Check sheet for the modelled part. Datum: model origin and axes. Units: mm. A direction names the side the tool comes from. Round coordinates to 2 decimals unless told otherwise and drop trailing zeros. Write each loop counter-clockwise with the first axis right and the second up, starting at its lowest first coordinate (ties: lowest second). Pieces come first, ordered by that corner, then holes.
Item 1: Section check A-A, the plane x = -7.75. Record the cut outline in (y, z).
Item 2: Release check for a two-part mould opening along X. For faces 1 (the cylindrical face through (-14.1, 49.3, 14.14)), 2 (the flat face through (0, 49, 13)), 3 (the flat face through (14, 0, 0)), 4 (the cylindrical face through (14.1, 49.3, -14.14)) record: pulls with the +X half, pulls with the -X half, needs draft (parallel to the pull), parting line crosses it, or undercut.
Item 3: Section check B-B, the plane z = 4.5. Record the cut outline in (x, y).
Item 4: Material ranges on line 1 along X through (y, z) = (61.5, 7.5); line 2 along Z through (x, y) = (12.5, 78), recorded low to high.
Item 5: Set-up check for faces 5 (the flat face through (0, 49, 15)), 6 (the flat face through (-13, 49, 0)): record each of +Z, -Z, +X, -X, +Y, -Y from which the full face is reachable in a straight line by a thin tool's end or side.
Item 6: Section check C-C, the plane y = 87. Record the cut outline in (x, z), plus the area to 3 significant figures.
Autodesk Inventor part; units mm, degrees
ref_plane "YZ Plane" through (0, 0, 0) normal (1, 0, 0) x (0, 1, 0)
ref_plane "XZ Plane" through (0, 0, 0) normal (0, 1, 0) x (-1, 0, 0)
ref_plane "XY Plane" through (0, 0, 0) normal (0, 0, 1) x (1, 0, 0)
sketch "Sketch1" plane through (0, 0, 0) normal (0, 1, 0) x (-1, 0, 0)
  line L0 (-12, 14) -> (12, 14) construction
  line L1 (14, 12) -> (14, -12) construction
  line L2 (12, -14) -> (-12, -14) construction
  line L3 (-14, -12) -> (-14, 12) construction
  line L4 (-14, 14) -> (14, -14) construction
  line L5 (14, 14) -> (-14, -14) construction
  arc A0 (14, 12) -> (12, 14) centre (12, 12) ccw construction
  arc A1 (12, -14) -> (14, -12) centre (12, -12) ccw construction
  arc A2 (-14, -12) -> (-12, -14) centre (-12, -12) ccw construction
  arc A3 (-12, 14) -> (-14, 12) centre (-12, 12) ccw construction
  line L6 (-12, -15) -> (12, -15)
  arc A4 (12, -15) -> (15, -12) centre (12, -12) ccw
  line L7 (15, -12) -> (15, 12)
  arc A5 (15, 12) -> (12, 15) centre (12, 12) ccw
  line L8 (12, 15) -> (-12, 15)
  arc A6 (-12, 15) -> (-15, 12) centre (-12, 12) ccw
  line L9 (-15, 12) -> (-15, -12)
  arc A7 (-15, -12) -> (-12, -15) centre (-12, -12) ccw
  line L10 (13, -12) -> (13, 12)
  arc A8 (13, 12) -> (12, 13) centre (12, 12) ccw
  line L11 (12, 13) -> (-12, 13)
  arc A9 (-12, 13) -> (-13, 12) centre (-12, 12) ccw
  line L12 (-13, 12) -> (-13, -12)
  arc A10 (-13, -12) -> (-12, -13) centre (-12, -12) ccw
  line L13 (-12, -13) -> (12, -13)
  arc A11 (12, -13) -> (13, -12) centre (12, -12) ccw
  point P0 (0, 0)
  point P1 (0, 0)
  point P2 (0, 0)
  dimension "d10" = 2
  dimension "depth" = 30
  dimension "width" = 30
  dimension "thickness" = 2
extrude "Extrusion1" add sketch "Sketch1" along normal blind 100
equation "\"d10\" = thickness"
properties part number "beam 30x30x2" material "Steel"
Values found:
1. outline: (0, -15) - (100, -15) - (100, -13) - (0, -13) - close; (0, 13) - (100, 13) - (100, 15) - (0, 15) - close
2. face 1: pulls with the -X half
2. face 2: undercut
2. face 3: needs draft
2. face 4: pulls with the +X half
3. outline: (-15, 0) - (-13, 0) - (-13, 100) - (-15, 100) - close; (13, 0) - (15, 0) - (15, 100) - (13, 100) - close
4. line 1: x = -15 to -13, 13 to 15
4. line 2: z = -14.96 to -12.87, 12.87 to 14.96
5. face 5: +Z, +X, -X, +Y, -Y
5. face 6: +Y, -Y
6. outline: (-15, -12) arc R3 ccw to (-12, -15) - (12, -15) arc R3 ccw to (15, -12) - (15, 12) arc R3 ccw to (12, 15) - (-12, 15) arc R3 ccw to (-15, 12) - close; hole (-13, -12) arc R1 ccw to (-12, -13) - (12, -13) arc R1 ccw to (13, -12) - (13, 12) arc R1 ccw to (12, 13) - (-12, 13) arc R1 ccw to (-13, 12) - close
6. area: 217 mm2
